Input: dimensioned drawing with shaded views. Units: mm. Origin: part minimum x, y, z. Coordinates: 2 decimals unless noted, no trailing zeros. Loops run counter-clockwise (first coordinate to the right, second up) from the corner with the lowest first, then second, coordinate; pieces in that order, holes last.
(1) Mould query, pull axis X, two halves, no side actions, for the marked faces 1, 2 and 3. Classes: released by +X, released by -X, zero draft, split by the parting line, or undercut.
(2) Section A-A, the plane y = 7.5. Return loops of the section in (x, z), then the cut area to 3 significant figures.
(3) Section B-B, the plane x = 12.5. Return loops of the section in (y, z), then the cut area to 3 significant figures.
(4) Line query: L1, parallel to Z at x = 2.5, y = 0.5. Output: solid intervals per line, ascending.
(5) Contact query for a flat-ended pin moving along its axis: P1, Ø4, axis at x = 5, y = 6.5, coming from the -Z side. Output: stop coordinate, or through.
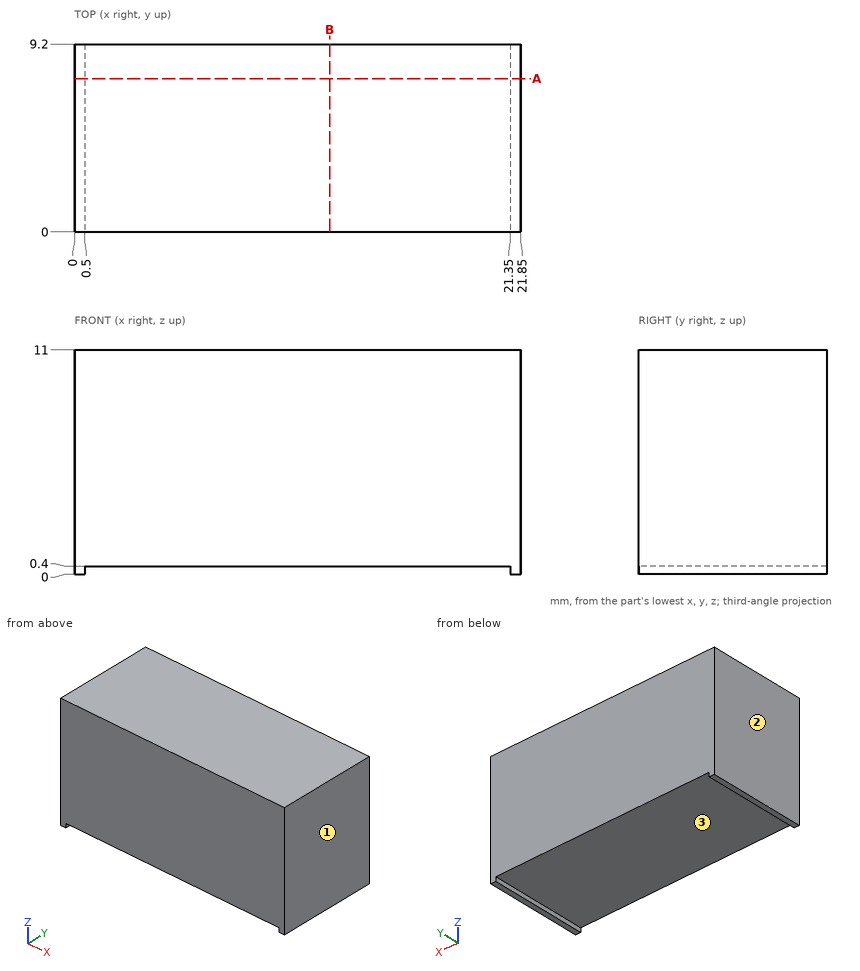
Report:
1. face 1: released by +X
1. face 2: released by -X
1. face 3: undercut
2. outline: (0, 0) - (0.5, 0) - (0.5, 0.4) - (21.35, 0.4) - (21.35, 0) - (21.85, 0) - (21.85, 11) - (0, 11) - close
2. area: 232 mm2
3. outline: (0, 0.4) - (9.2, 0.4) - (9.2, 11) - (0, 11) - close
3. area: 97.5 mm2
4. L1: z = 0.4 to 11
5. P1: stops at z = 0.4
